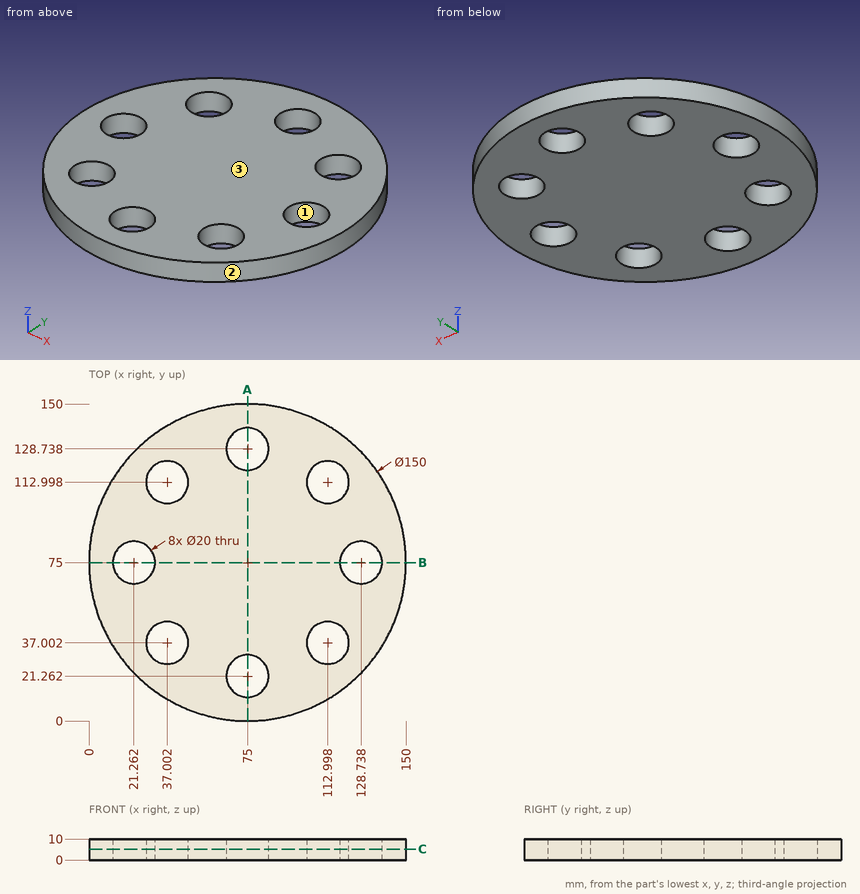
Could you check a few things on this drawing? It's one solid part, dimensions in mm from its lowest x, y, z. Coordinates: 2 decimals unless noted, no trailing zeros. Write each loop counter-clockwise with the first axis right and the second up, starting at its lowest first coordinate (ties: lowest second). Pieces come first, ordered by that corner, then holes.
1) Thinking about a two-plate mould opening in Y: for the marked faces 1, 2 and 3, which applies, +Y half, -Y half, draft (parallel to the pull), parting line (faces both ways), or undercut?
Filled in:
face 1: undercut
face 2: parting line
face 3: draft
2) I'm going to push flat-ended pins straight in: pin 1 (18 mm diameter, centred on x = 75, y = 128.74, fed in from -Z); pin 2 (12 mm diameter, centred on x = 50, y = 91, fed in from -Z); pin 3 (1 mm diameter, centred on x = 102, z = 7.5, fed in from +Y); pin 4 (4 mm diameter, centred on x = 52, z = 3, fed in from +Y). Where does each tip first touch, or does it pass through?
Filled in:
pin 1: passes through
pin 2: stops at z = 0
pin 3: stops at y = 145.16
pin 4: stops at y = 147
3) If we section it at C-C (z = 5.25): Count the separate pieces of the cut face and the enclosed holes in it, plus the area to 3 significant figures.
Filled in:
separate pieces: 1
enclosed holes: 8
area: 15,200 mm2
4) If we section it at A-A (x = 75): List the corners of the cut face in (y, z) for me, plus the area to 3 significant figures.
Filled in:
outline: (0, 0) - (11.26, 0) - (11.26, 10) - (0, 10) - close; (31.26, 0) - (118.74, 0) - (118.74, 10) - (31.26, 10) - close; (138.74, 0) - (150, 0) - (150, 10) - (138.74, 10) - close
area: 1,100 mm2
5) If I drill on line 1 (Y direction, x = 75, z = 3.5); line 2 (Y direction, x = 38.5, z = 3.5) (1 decimal); line 3 (X direction, y = 110.5, z = 1) (1 decimal), over which ranges is the centre line in solid material (lowest first)?
Filled in:
line 1: y = 0 to 11.26, 31.26 to 118.74, 138.74 to 150
line 2: y = 9.5 to 27.1, 46.9 to 103.1, 122.9 to 140.5
line 3: x = 8.9 to 27.3, 46.7 to 103.3, 122.7 to 141.1
